from build123d import *

# Parameters (mm, degrees)
F0_W          = 2724.15
F0_H          = 419.1
F1_DEPTH      = 609.6
F3_DEPTH      = 1362.076
F3_DEPTH_BACK = 1362.076
F4_W          = 25.4
F4_H          = 571.5
F5_DEPTH      = 419.101
F7_DEPTH      = 419.101
F8_W          = 609.6
F8_H          = 215.9
F9_DEPTH      = 2.54
F11_DEPTH     = 393.7
F12_W         = 2724.15
F12_H         = 38.1
F13_DEPTH     = 25.4


with BuildPart() as f1:
    # F0 (on Top) → F1 (new body)
    with BuildSketch(Plane.XY):
        with Locations((0, -209.55)):
            Rectangle(F0_W, F0_H)
    extrude(amount=-F1_DEPTH)

    # F2 (on Right) → F3 (cut, two sides)
    with BuildSketch(Plane.YZ) as f3_sk:
        Polygon((-101.6, -419.1), (-101.6, -609.6), (0, -609.6), (0, -368.3), (-50.8, -368.3), align=None)
    extrude(amount=F3_DEPTH, mode=Mode.SUBTRACT)
    extrude(f3_sk.sketch, amount=-F3_DEPTH_BACK, mode=Mode.SUBTRACT)

    # F4 (on face) → F5 (cut, through all)
    with BuildSketch(Plane.XZ.offset(419.1)):
        with Locations((1349.375, -323.85)):
            Rectangle(F4_W, F4_H)
        with Locations((-1349.375, -323.85)):
            Rectangle(F4_W, F4_H)
    extrude(amount=-F5_DEPTH, mode=Mode.SUBTRACT)

    # F6 (on face) → F7 (cut, through all)
    with BuildSketch(Plane.XZ.offset(419.1)):
        Polygon((-1260.475, -431.8), (-1260.475, -609.6), (-38.1, -609.6), (-38.1, -431.8), (-114.3, -355.6), (-1184.275, -355.6), align=None)
        Polygon((38.1, -431.8), (38.1, -609.6), (1158.875, -609.6), (1158.875, -431.8), (1082.675, -355.6), (114.3, -355.6), align=None)
        Polygon((1235.075, -431.8), (1235.075, -609.6), (1336.675, -609.6), (1336.675, -355.6), (1311.275, -355.6), align=None)
    extrude(amount=-F7_DEPTH, mode=Mode.SUBTRACT)

    # F8 (on face) → F9 (join)
    with BuildSketch(Plane.XZ.offset(419.1)):
        with Locations((-984.885, -146.05)):
            Rectangle(F8_W, F8_H)
        with Locations((-328.295, -146.05)):
            Rectangle(F8_W, F8_H)
        with Locations((328.295, -146.05)):
            Rectangle(F8_W, F8_H)
        with Locations((984.885, -146.05)):
            Rectangle(F8_W, F8_H)
    extrude(amount=F9_DEPTH)

    # F10 (on face) → F11 (cut, through all)
    with BuildSketch(Plane(origin=(0, 0, 0), x_dir=(-1, 0, 0), z_dir=(0, 1, 0))):
        Polygon((-1184.275, -609.6), (-1209.675, -609.6), (-1209.675, -279.4), (-1336.675, -279.4), (-1336.675, -635), (1336.675, -635), (1336.675, -279.4), (1311.275, -279.4), (1311.275, -609.6), (1285.875, -609.6), (1285.875, -279.4), (12.7, -279.4), (12.7, -609.6), (-12.7, -609.6), (-12.7, -279.4), (-1184.275, -279.4), align=None)
    extrude(amount=-F11_DEPTH, mode=Mode.SUBTRACT)

    # F12 (on face) → F13 (join)
    with BuildSketch(Plane.XZ.offset(419.1)):
        with Locations((0, -19.05)):
            Rectangle(F12_W, F12_H)
    extrude(amount=F13_DEPTH)


solid = f1.part
Geometry: final body of the model. Coordinates: model frame, mm. A direction names the side the tool comes from. Coordinates: 2 decimals unless noted, no trailing zeros. Order: outer loops, then holes, each group sorted by start corner. A loop starts at its lowest first (then second) coordinate and runs counter-clockwise, first axis right, second up. Notation, with made-up numbers: M -17,-21.75 L 37,-21.75 A20 ccw 37,-2.75 Z; hole C -24.5,-14 d5. An arc over 180 degrees is marked long. One line per question, with ' | ' between items. Start each with the question number.
Item 1: Set-up query: faces 1 (the flat face through (1260, -393.7, -369)), 2 (the flat face through (601, -393.7, -346)), 3 (the flat face through (-1311.275, -238, -442)), 4 (the flat face through (-989, -421.64, -145)), 5 (the flat face through (1336.675, -212, -164)). Return all of +Z, -Z, +X, -X, +Y, -Y with unobstructed straight access to the full face (end or side cutting, diameter ignored); none if empty.
Item 2: Pin query (flat end, axial travel): pin 1 Ø20.5 at (x, y) = (384, -412) entering from -Z; pin 2 Ø1.3 at (x, y) = (-215, -421) entering from -Z; pin 3 Ø4 at (y, z) = (-250, -307.5) entering from +X (3 decimals); pin 4 Ø5 at (x, y) = (-10.5, -377.5) entering from +Z. Return the tip coordinate at first contact, or that it passes through.
Item 3: Cut plane A-A, the plane z = -546.5. Return the cut outline in (x, y) (3 decimals), then the cut area to 3 significant figures.
Item 4: Cut plane D-D, the plane x = 776. Return the cut outline in (y, z).
Item 5: Cut plane C-C, the plane z = -141.5. Return the cut outline in (x, y) (3 decimals).
Item 6: Ray query, probe 1 along X at (y, z) = (-154.5, -311) (3 decimals); probe 2 along Z at (x, y) = (1237.5, -127); probe 3 along Y at (x, z) = (-36.5, -495.5). Return the intervals inside material, ascending. Write a range as [from, to].
Item 7: Cut plane B-B, the plane y = -348. Return the cut outline in (x, z) (3 decimals), then the cut area to 3 significant figures.
A:
1) face 1: -Z, +X, +Y | face 2: -Z, +Y | face 3: -Z, -X, +Y | face 4: -Z, +X, -X, -Y | face 5: -Z, +X, +Y, -Y
2) pin 1: stops at z = -355.6 | pin 2: stops at z = -254 | pin 3: stops at x = 1209.675 | pin 4: stops at z = 0
3) outline: M -1336.675,-419.1 L -1260.475,-419.1 L -1260.475,-393.7 L -1285.875,-393.7 L -1285.875,-101.6 L -1311.275,-101.6 L -1311.275,-393.7 L -1336.675,-393.7 Z; M -38.1,-419.1 L 38.1,-419.1 L 38.1,-393.7 L 12.7,-393.7 L 12.7,-101.6 L -12.7,-101.6 L -12.7,-393.7 L -38.1,-393.7 Z; M 1158.875,-419.1 L 1235.075,-419.1 L 1235.075,-393.7 L 1209.675,-393.7 L 1209.675,-101.6 L 1184.275,-101.6 L 1184.275,-393.7 L 1158.875,-393.7 Z | area: 28,100 mm2
4) outline: M -444.5,-38.1 L -421.64,-38.1 L -421.64,-254 L -419.1,-254 L -419.1,-355.6 L -393.7,-355.6 L -393.7,-279.4 L 0,-279.4 L 0,0 L -444.5,0 Z
5) outline: M -1336.675,-419.1 L -1289.685,-419.1 L -1289.685,-421.64 L -680.085,-421.64 L -680.085,-419.1 L -633.095,-419.1 L -633.095,-421.64 L -23.495,-421.64 L -23.495,-419.1 L 23.495,-419.1 L 23.495,-421.64 L 633.095,-421.64 L 633.095,-419.1 L 680.085,-419.1 L 680.085,-421.64 L 1289.685,-421.64 L 1289.685,-419.1 L 1336.675,-419.1 L 1336.675,0 L -1336.675,0 Z
6) probe 1: x = [-1311.275, -1285.875], [-12.7, 12.7], [1184.275, 1209.675] | probe 2: z = [-279.4, 0] | probe 3: y = [-419.1, -393.7]
7) outline: M -1362.075,-38.1 L -1336.675,-38.1 L -1336.675,-279.4 L -1311.275,-279.4 L -1311.275,-609.6 L -1285.875,-609.6 L -1285.875,-279.4 L -12.7,-279.4 L -12.7,-609.6 L 12.7,-609.6 L 12.7,-279.4 L 1184.275,-279.4 L 1184.275,-609.6 L 1209.675,-609.6 L 1209.675,-279.4 L 1336.675,-279.4 L 1336.675,-38.1 L 1362.075,-38.1 L 1362.075,0 L -1362.075,0 Z | area: 774,000 mm2
